Part model, mm, in its own coordinate system. A direction names the side the tool comes from. Coordinates: 2 decimals unless noted, no trailing zeros. Loops run counter-clockwise (first coordinate to the right, second up) from the corner with the lowest first, then second, coordinate; pieces in that order, holes last. Notation, with made-up numbers: (52.25, 48) -> (70.25, 48) arc R10 cw to (70.25, 54) -> close; hole circle Ø4 at (80.5, 67.5). An arc over 180 degrees is marked (long way). Use one line per item in the form item = value. Start each with the question number.
(1) Pin check, flat tip, straight feed: P1, Ø4, axis at y = -34.5, z = -6, coming from the +X side. Stop position of the tip, or through.
(2) 3-axis set-ups, long thin cutter, end or side, ignore diameter. For faces 1 (the flat face through (-19.812, -47, -9)), 2 (the cylindrical face through (-26.527, -28.704, -9.392)): which of +Z, -Z, +X, -X, +Y, -Y reach the whole face in a straight line?
(3) Drill centre lines: L1, parallel to Z at x = -25.75, y = -41.25; L2, parallel to Y at x = -23.5, z = -8.75; L3, parallel to X at y = -42.5, z = -10. Where is each one in solid material? Low to high. Write a range as [from, to].
(4) Band-saw the part on D-D on x = -21.75. Give the cut face in (y, z).
(5) Mould opens along Z. For faces 3 (the cylindrical face through (-28.232, -25.338, -9.356)), 4 (the flat face through (-24, -27.75, -9)), 5 (the flat face through (-24, -36, -21.59)) say: +Z half, -Z half, draft (parallel to the pull), parting line (faces both ways), or undercut.
(6) Band-saw the part on B-B on y = -33.5. Give the cut face in (x, z).
(7) Band-saw the part on A-A on x = -23.75. Give the cut face in (y, z), then the cut area to 3 significant figures.
```python
from build123d import *

# Parameters (mm, degrees)
BOSS_EXTRUDE1_DEPTH = 19.05
BOSS_EXTRUDE2_START = 2.54
BOSS_EXTRUDE2_DEPTH = 2.54
BOSS_EXTRUDE3_DEPTH = 2.54
FILLET1_R           = 2.54


with BuildPart() as part:
    # Sketch1 → Boss-Extrude1 (new body)
    with BuildSketch(Plane.XY):
        with BuildLine():
            ThreePointArc((-22.987, -27.7495), (-20.74193597, -26.81956403), (-19.812, -24.5745))
            Line((-19.812, -24.5745), (-28.956, -24.5745))
            Line((-28.956, -24.5745), (-28.956, -48.7045))
            Line((-28.956, -48.7045), (-19.812, -48.7045))
            Line((-19.812, -48.7045), (-19.812, -46.7995))
            Line((-19.812, -46.7995), (-24.257, -46.7995))
            ThreePointArc((-24.257, -46.7995), (-26.50206403, -45.86956403), (-27.432, -43.6245))
            Line((-27.432, -43.6245), (-27.432, -30.9245))
            ThreePointArc((-27.432, -30.9245), (-26.50206403, -28.67943597), (-24.257, -27.7495))
            Line((-24.257, -27.7495), (-22.987, -27.7495))
        make_face()
    extrude(amount=-BOSS_EXTRUDE1_DEPTH)

    # Sketch2 → Boss-Extrude2 (add)
    with BuildSketch(Plane.XY.offset(BOSS_EXTRUDE2_START)):
        with BuildLine():
            Line((-19.812, -46.7995), (-24.257, -46.7995))
            ThreePointArc((-24.257, -46.7995), (-26.50206403, -45.86956403), (-27.432, -43.6245))
            Line((-27.432, -43.6245), (-27.432, -30.9245))
            ThreePointArc((-27.432, -30.9245), (-26.50206403, -28.67943597), (-24.257, -27.7495))
            Line((-24.257, -27.7495), (-22.987, -27.7495))
            ThreePointArc((-22.987, -27.7495), (-20.74193597, -26.81956403), (-19.812, -24.5745))
            Line((-19.812, -24.5745), (-28.956, -24.5745))
            Line((-28.956, -24.5745), (-28.956, -48.7045))
            Line((-28.956, -48.7045), (-19.812, -48.7045))
            Line((-19.812, -48.7045), (-19.812, -46.7995))
        make_face()
        with BuildLine():
            Line((-19.812, -46.7995), (-19.812, -24.5745))
            ThreePointArc((-19.812, -24.5745), (-20.74193597, -26.81956403), (-22.987, -27.7495))
            Line((-22.987, -27.7495), (-24.257, -27.7495))
            ThreePointArc((-24.257, -27.7495), (-26.50206403, -28.67943597), (-27.432, -30.9245))
            Line((-27.432, -30.9245), (-27.432, -43.6245))
            ThreePointArc((-27.432, -43.6245), (-26.50206403, -45.86956403), (-24.257, -46.7995))
            Line((-24.257, -46.7995), (-19.812, -46.7995))
        make_face()
    extrude(amount=-BOSS_EXTRUDE2_DEPTH)

    # Sketch3 → Boss-Extrude3 (add)
    with BuildSketch(Plane(origin=(0, 0, -19.05), x_dir=(-1, 0, 0), z_dir=(0, 0, -1))):
        with BuildLine():
            ThreePointArc((22.987, -27.7495), (20.74193597, -26.81956403), (19.812, -24.5745))
            Line((19.812, -24.5745), (19.812, -46.7995))
            Line((19.812, -46.7995), (24.257, -46.7995))
            ThreePointArc((24.257, -46.7995), (26.50206403, -45.86956403), (27.432, -43.6245))
            Line((27.432, -43.6245), (27.432, -30.9245))
            ThreePointArc((27.432, -30.9245), (26.50206403, -28.67943597), (24.257, -27.7495))
            Line((24.257, -27.7495), (22.987, -27.7495))
        make_face()
        with BuildLine():
            Line((27.432, -30.9245), (27.432, -43.6245))
            ThreePointArc((27.432, -43.6245), (26.50206403, -45.86956403), (24.257, -46.7995))
            Line((24.257, -46.7995), (19.812, -46.7995))
            Line((19.812, -46.7995), (19.812, -48.7045))
            Line((19.812, -48.7045), (28.956, -48.7045))
            Line((28.956, -48.7045), (28.956, -24.5745))
            Line((28.956, -24.5745), (19.812, -24.5745))
            ThreePointArc((19.812, -24.5745), (20.74193597, -26.81956403), (22.987, -27.7495))
            Line((22.987, -27.7495), (24.257, -27.7495))
            ThreePointArc((24.257, -27.7495), (26.50206403, -28.67943597), (27.432, -30.9245))
        make_face()
    extrude(amount=BOSS_EXTRUDE3_DEPTH)

    # Fillet1
    fillet1_edges = [part.edges().sort_by_distance(p)[0] for p in [
        (-28.956, -48.7045, -9.525),
        (-28.956, -24.5745, -9.525),
    ]]
    fillet(fillet1_edges, radius=FILLET1_R)


solid = part.part
```
A:
q1.P1 = -27.43
q2.face_1 = +Z, -Z, +X, +Y, -Y
q2.face_2 = +X
q3.L1 = [-21.59, -19.05], [0, 2.54]
q3.L2 = [-48.7, -46.8], [-27.75, -24.57]
q3.L3 = [-28.96, -27.43]
q4.outline = (-48.7, -21.59) -> (-24.57, -21.59) -> (-24.57, 2.54) -> (-48.7, 2.54) -> close; hole (-46.8, -19.05) -> (-27.5, -19.05) -> (-27.5, 0) -> (-46.8, 0) -> close
q5.face_3 = draft
q5.face_4 = undercut
q5.face_5 = -Z half
q6.outline = (-28.96, -21.59) -> (-19.81, -21.59) -> (-19.81, -19.05) -> (-27.43, -19.05) -> (-27.43, 0) -> (-19.81, 0) -> (-19.81, 2.54) -> (-28.96, 2.54) -> close
q7.outline = (-48.7, -21.59) -> (-24.57, -21.59) -> (-24.57, 2.54) -> (-48.7, 2.54) -> close; hole (-46.8, -19.05) -> (-27.75, -19.05) -> (-27.75, 0) -> (-46.8, 0) -> close
q7.area = 219 mm²
